Geometry: final body of the model. Coordinates: model frame, mm. Face numbers are marked on the shaded views. A direction names the side the tool comes from. Coordinates: 2 decimals unless noted, no trailing zeros. Order: outer loops, then holes, each group sorted by start corner. A loop starts at its lowest first (then second) coordinate and runs counter-clockwise, first axis right, second up. Notation, with made-up numbers: M 82,13.5 L 99,13.5 A32 ccw 99,50.5 Z; hole C 1.5,-7 d5. An arc over 180 degrees is marked long. Use CSV: the item, a comma, the result in double quotes. Start each with the question number.
1. Section query C-C on x = 19. Return the cut outline in (y, z), and give its area (3 significant figures).
2. Material intervals for line 1 (Z direction, x = -14, y = 0.5); line 2 (Y direction, x = 6, z = 21.5); line 3 (X direction, y = 7, z = -2), sorted ascending.
3. First-contact query: P1, Ø4, axis at x = 6, y = 8, coming from the +Z side; P2, Ø5, axis at x = 8, z = -8, coming from the -Y side; P3, Ø3, axis at x = 12.5, z = -16.23, coming from the +Y side; P4, Ø2.5, axis at y = 7, z = -5.5, coming from the +X side. Flat tips, straight axial feed; report the tip coordinate or a pass-through.
4. Section query B-B on y = 7.5. Return the cut outline in (x, z).
5. Section query A-A on z = 3.5. Return the cut outline in (x, y).
6. Set-up query: the marked faces 1 and 2. Return all of +Z, -Z, +X, -X, +Y, -Y with unobstructed straight access to the full face (end or side cutting, diameter ignored); none if empty.
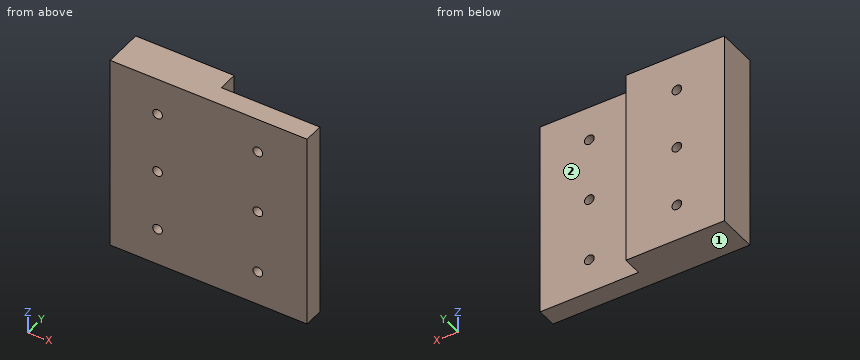
Autodesk Inventor part; units mm, degrees
ref_plane "YZ Plane" through (0, 0, 0) normal (1, 0, 0) x (0, 1, 0)
ref_plane "XZ Plane" through (0, 0, 0) normal (0, 1, 0) x (-1, 0, 0)
ref_plane "XY Plane" through (0, 0, 0) normal (0, 0, 1) x (1, 0, 0)
sketch "Sketch1" plane through (0, 0, 0) normal (0, 1, 0) x (-1, 0, 0)
  line L0 (25, 25) -> (-25, 25)
  line L1 (-25, 25) -> (-25, -25)
  line L2 (-25, -25) -> (25, -25)
  line L3 (25, -25) -> (25, 25)
  line L4 (35, 0) -> (-35, 0)
  line L5 (0, -35) -> (0, 35)
  point P0 (0, 0)
  dimension "d0" = 50
  dimension "d1" = 50
extrude "Extrusion1" add sketch "Sketch1" along normal blind 10
sketch "Sketch2" plane through (0, 10, 0) normal (0, 1, 0) x (1, 0, 0)
  line L0 (-25, -25) -> (25, -25)
  line L1 (25, -25) -> (25, 25)
  line L2 (0, -25) -> (25, -25)
  line L3 (25, -25) -> (25, 25)
  line L4 (25, 25) -> (0, 25)
  line L5 (0, 25) -> (0, -25)
  point P0 (0, 0)
extrude "Extrusion2" cut sketch "Sketch2" against normal blind 5
sketch "Sketch3" plane through (0, 10, 0) normal (0, 1, 0) x (1, 0, 0)
  line L0 (-12.9579, -25.0914) -> (-12.9579, 25) construction
  line L1 (25, 25) -> (-25, 25) construction
  line L2 (12.5042, -25.0914) -> (12.5042, 25) construction
  line L3 (-35, 0) -> (35, 0) construction
  point P0 (0, 0)
  point P1 (-12.9579, -0.0457)
  point P2 (-12.9579, -15.5571)
  point P3 (-12.9579, 15.5571)
  point P4 (12.5042, -16.2302)
  point P5 (12.5042, -0.0457)
  point P6 (12.5042, 16.2302)
hole "Hole1" at (-12.9579, 10, 0.0457) at (-12.9579, 10, -15.5571) at (12.5042, 10, 16.2302) at (12.5042, 10, 0.0457) at (12.5042, 10, -16.2302) at (-12.9579, 10, 15.5571) direction (0, -1, 0) diameter 2.459 depth 10
equation "\"d1\" = d0"
properties part number "screwbase"
Results list:
1,outline,"M 0,-25 L 5,-25 L 5,25 L 0,25 Z"
1,area,"250 mm²"
2,line 1,"z = -25 to -16.21, -14.9 to -0.61, 0.7 to 14.9, 16.21 to 25"
2,line 2,"y = 0 to 5"
2,line 3,"x = -25 to 0"
3,P1,"passes through"
3,P2,"stops at y = 0"
3,P3,"stops at y = 5"
3,P4,"stops at x = 0"
4,outline,"M -25,-25 L 0,-25 L 0,25 L -25,25 Z; hole C -12.96,-15.56 d2.46; hole C -12.96,0.05 d2.46; hole C -12.96,15.56 d2.46"
5,outline,"M -25,0 L 25,0 L 25,5 L 0,5 L 0,10 L -25,10 Z"
6,face 1,"-Z, +X, -X, +Y, -Y"
6,face 2,"+Z, -Z, +X, +Y"
